Work out the finished part from the listing and answer in its coordinate system (mm). Face numbers are marked on the shaded views. A direction names the side the tool comes from. Coordinates: 2 decimals unless noted, no trailing zeros. Write each loop counter-clockwise with the first axis right and the second up, starting at its lowest first coordinate (ties: lowest second). Pieces come first, ordered by that corner, then holes. Notation, with made-up numbers: M 23.25,78.5 L 61.25,78.5 A14 ccw 61.25,99.5 Z; hole C 35,50.25 d9. An arc over 180 degrees is marked long. Answer as CSV lines item,"result". Start each with the question number.
(1) The mould has two halves that part along X. Classify the marked faces 4, 5 and 6: released by +X, released by -X, zero draft, split by the parting line, or undercut.
(2) A cutting plane is placed at B-B on y = -4.25. Give the vertices of the cut face in (x, z).
(3) A cutting plane is placed at A-A on x = 38.5. Give the vertices of the cut face in (y, z), then the cut area to 3 significant figures.
(4) Find the intervals of material crossed by L1, parallel to X at y = 6, z = 1.75; L2, parallel to X at y = 3.25, z = 0.5; L3, parallel to Y at x = 13, z = -4, in increasing order. Write a range as [from, to].
(5) A cutting plane is placed at D-D on y = 4. Give the vertices of the cut face in (x, z).
(6) For the marked faces 1, 2 and 3, determine the directions among +Z, -Z, +X, -X, +Y, -Y from which every point of the face is accessible in a straight line to the end or side of a thin tool.
(7) Flat-ended cylindrical pins translate along their axes: P1, Ø6.5, axis at y = 0.5, z = 0.5, coming from the +X side; P2, Ø1.5, axis at y = 3, z = -4.5, coming from the -X side; P3, Ø4, axis at y = -1.5, z = 5, coming from the +X side; P4, Ø6, axis at x = 7.5, y = 4.5, coming from the +Z side. Find the tip coordinate at first contact, or state that the pin passes through.
(8) A cutting plane is placed at C-C on x = 11.5. Give the vertices of the cut face in (y, z).
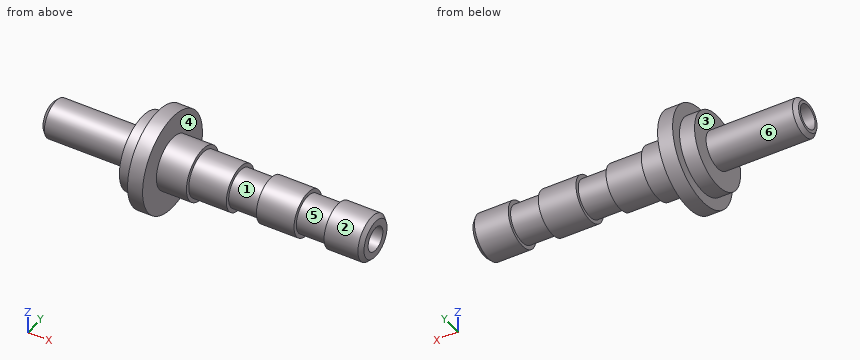
from build123d import *

# Parameters (mm, degrees)
F2_R     = 1.6
F3_DEPTH = 43.001
F4_SIZE  = 0.5


with BuildPart() as f1:
    # F0 (on Front) → F1 (revolve)
    with BuildSketch(Plane.XZ):
        Polygon((0, 2.5), (0, 0), (43, 0), (43, 3), (38, 3), (38, 2.5), (34, 2.5), (34, 3), (29, 3), (29, 2.5), (25, 2.5), (25, 3), (20, 3), (20, 3.5), (16, 3.5), (16, 6.5), (14, 6.5), (14, 5), (12, 5), (12, 2.5), align=None)
    revolve(axis=Axis((-2.710388, 0, 0), (-1, 0, 0)))

    # F2 (on face) → F3 (cut, through all)
    with BuildSketch(Plane.YZ.offset(43)):
        Circle(F2_R)
    extrude(amount=-F3_DEPTH, mode=Mode.SUBTRACT)

    # F4
    f4_edges = [f1.edges().sort_by_distance(p)[0] for p in [
        (43, 0, -3),
        (0, 0, -2.5),
    ]]
    chamfer(f4_edges, length=F4_SIZE)


solid = f1.part
Here are the results:
1,face 4,"released by +X"
1,face 5,"undercut"
1,face 6,"zero draft"
2,outline,"M 12,-2.63 L 14,-2.63 L 14,-4.92 L 16,-4.92 L 16,4.92 L 14,4.92 L 14,2.63 L 12,2.63 Z"
3,outline,"C 0,0 d6; hole C 0,0 d3.2"
3,area,"20.2 mm^2"
4,L1,"x = [14, 16]"
4,L2,"x = [12, 20]"
4,L3,"y = [-3, 3]"
5,outline,"M 12,-3 L 14,-3 L 14,-5.12 L 16,-5.12 L 16,5.12 L 14,5.12 L 14,3 L 12,3 Z"
6,face 1,"none"
6,face 2,"+X"
6,face 3,"-X"
7,P1,"stops at x = 43"
7,P2,"stops at x = 12"
7,P3,"stops at x = 20"
7,P4,"stops at z = 2"
8,outline,"C 0,0 d5; hole C 0,0 d3.2"
